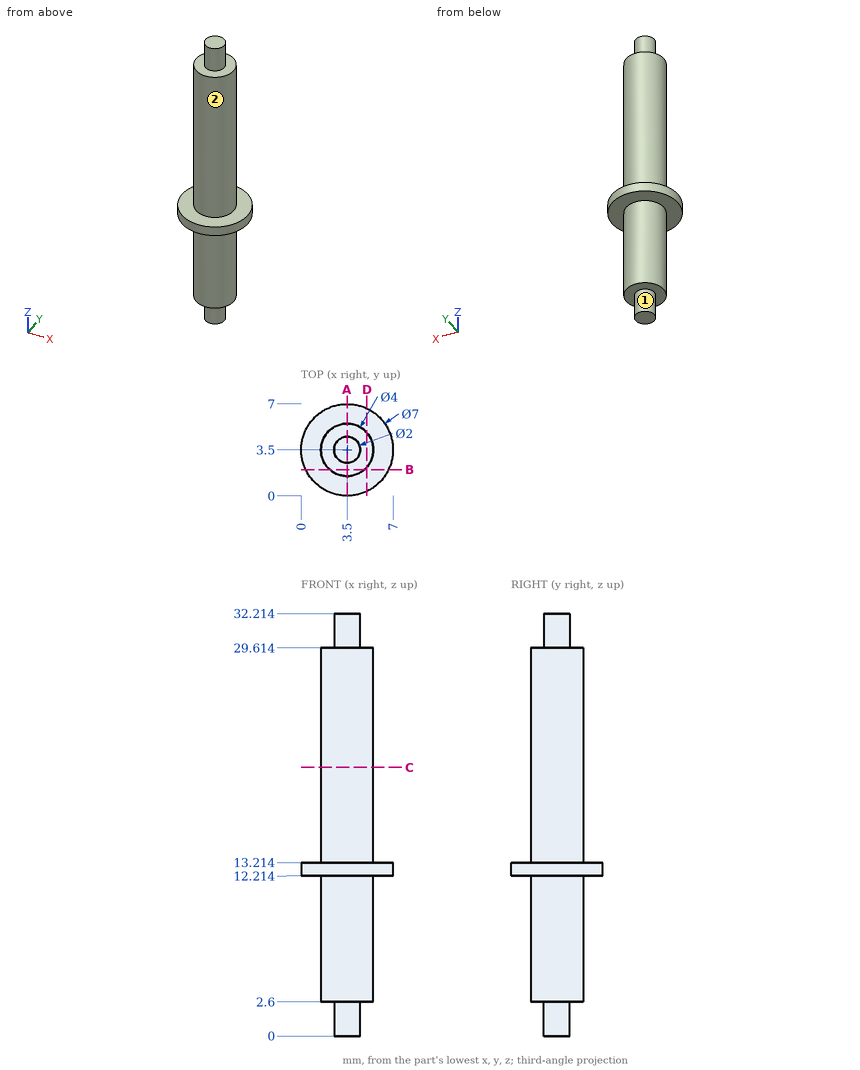
Can you work these out from the drawing? Everything is in mm from the part's minimum corner. A direction names the side the tool comes from. Give positions to 0.01 mm unless a question says otherwise; leave off trailing zeros. Loops run counter-clockwise (first coordinate to the right, second up) from the corner with the lowest first, then second, coordinate; pieces in that order, holes last. Notation, with made-up numbers: (-36, -0.75) -> (16, -0.75) arc R11 cw to (16, 8.25) -> close; hole circle Ø5 at (-37, 78.25). An arc over 180 degrees is marked (long way). Return JSON: item names as keys, results as strings.
Item 1: If we section it at C-C on z = 20.5: List the corners of the cut face in (x, y) for me.
Geometry results:
{"outline": "circle Ø4 at (3.5, 3.5)"}
Item 2: If we section it at B-B on y = 2: List the corners of the cut face in (x, z) for me.
Geometry results:
{"outline": "(0.34, 12.21) -> (2.18, 12.21) -> (2.18, 2.6) -> (4.82, 2.6) -> (4.82, 12.21) -> (6.66, 12.21) -> (6.66, 13.21) -> (4.82, 13.21) -> (4.82, 29.61) -> (2.18, 29.61) -> (2.18, 13.21) -> (0.34, 13.21) -> close"}
Item 3: Which directions (+Z, -Z, +X, -X, +Y, -Y) give clear straight access to the entire face, cutting with the end or side of a thin tool? Please do the marked faces 1 and 2.
Geometry results:
{"face 1": "-Z", "face 2": "+Z"}
Item 4: I need wall thicknesses on L1, parallel to Z at x = 3, y = 1; L2, parallel to X at y = 3.5, z = 21; L3, parallel to Y at x = 4, z = 13 (1 decimal). Which ranges of each line are inside material? Lowest first, please. Write a range as from..to.
Geometry results:
{"L1": "z = 12.21..13.21", "L2": "x = 1.5..5.5", "L3": "y = 0..7"}
Item 5: If we section it at A-A on x = 3.5: List the corners of the cut face in (y, z) for me.
Geometry results:
{"outline": "(0, 12.21) -> (1.5, 12.21) -> (1.5, 2.6) -> (2.5, 2.6) -> (2.5, 0) -> (4.5, 0) -> (4.5, 2.6) -> (5.5, 2.6) -> (5.5, 12.21) -> (7, 12.21) -> (7, 13.21) -> (5.5, 13.21) -> (5.5, 29.61) -> (4.5, 29.61) -> (4.5, 32.21) -> (2.5, 32.21) -> (2.5, 29.61) -> (1.5, 29.61) -> (1.5, 13.21) -> (0, 13.21) -> close"}
Item 6: I'm going to push flat-ended pins straight in: pin 1 (2 mm diameter, centred on y = 1, z = 23, fed in from +X); pin 2 (1.5 mm diameter, centred on x = 2, y = 1.5, fed in from +Z); pin 3 (4 mm diameter, centred on y = 3, z = 12.5, fed in from -X). Where does each tip first touch, or does it pass through?
Geometry results:
{"pin 1": "stops at x = 4.82", "pin 2": "stops at z = 29.61", "pin 3": "stops at x = 0"}
